from build123d import *

# Parameters (mm, degrees)
SKETCH1_W           = 80
SKETCH1_H           = 80
BOSS_EXTRUDE1_DEPTH = 5
SKETCH2_W           = 10
SKETCH2_H           = 4.637634929
BOSS_EXTRUDE2_DEPTH = 7
SKETCH3_R           = 1.5
CUT_EXTRUDE1_DEPTH  = 91


with BuildPart() as part:
    # Sketch1 → Boss-Extrude1 (new body)
    with BuildSketch(Plane.XY):
        Polygon((-50, 40), (-45, 40), (-45, 50), (45, 50), (45, 40), (50, 40), (50, -40), (45, -40), (45, -50), (-45, -50), (-45, -40), (-50, -40), align=None)
        Rectangle(SKETCH1_W, SKETCH1_H, mode=Mode.SUBTRACT)
    extrude(amount=BOSS_EXTRUDE1_DEPTH)

    # Sketch2 → Boss-Extrude2 (add)
    with BuildSketch(Plane.XY.offset(5)):
        with Locations((45, -37.681182535)):
            Rectangle(SKETCH2_W, SKETCH2_H)
        with Locations((-45, -37.681182535)):
            Rectangle(SKETCH2_W, SKETCH2_H)
        with Locations((-45, 37.681182535)):
            Rectangle(SKETCH2_W, SKETCH2_H)
        with Locations((45, 37.681182535)):
            Rectangle(SKETCH2_W, SKETCH2_H)
    extrude(amount=BOSS_EXTRUDE2_DEPTH)

    # Sketch3 → Cut-Extrude1 (cut, through all)
    with BuildSketch(Plane.XZ.offset(40)):
        with Locations((-47.5, 8)):
            Circle(SKETCH3_R)
        with Locations((47.5, 8)):
            Circle(SKETCH3_R)
    extrude(amount=-CUT_EXTRUDE1_DEPTH, mode=Mode.SUBTRACT)


solid = part.part
CAD build for the part. Positions are in the model's coordinates, mm. A direction names the side the tool comes from. Give positions to 0.01 mm unless a question says otherwise; leave off trailing zeros. Loops run counter-clockwise (first coordinate to the right, second up) from the corner with the lowest first, then second, coordinate; pieces in that order, holes last. Notation, with made-up numbers: M -29,62.5 L -15,62.5 A6 cw -15,67.5 Z; hole C 12.25,-7.5 d5. An arc over 180 degrees is marked long. One line per question, with ' | ' between items. Start each with the question number.
1. Probe L1, parallel to Z at x = 47.5, y = 36.75; L2, parallel to Y at x = -44, z = 7.5; L3, parallel to Y at x = 0, z = 2.25. List the from-to ranges inside material, lowest first. Write a range as from..to.
2. Two-plate mould, pull along X, no slides. Class faces 1 (the face through (45, 45, 2)), 2 (the face through (46, -38, 8)), 3 (the face through (46, 38, 8)), 4 (the face through (-45, -38, 12)): pulls with the +X half, pulls with the -X half, needs draft (parallel to the pull), parting line crosses it, or undercut.
3. Flat gauge pins, fed straight in: pin 1 (8 mm diameter, centred on x = 45.5, y = -4.5, fed in from +Z); pin 2 (5.5 mm diameter, centred on x = -45.5, z = 9, fed in from +Y); pin 3 (2.5 mm diameter, centred on x = -47.5, z = 8, fed in from +Y); pin 4 (3 mm diameter, centred on x = 44, z = 7, fed in from -Y). Where does each tip first touch, or does it go through?
4. Saw through at B-B on y = -38.5. Give the cut face in (x, z), plus the area to 3 significant figures.
5. Saw through at D-D on x = -32.5. Give the cut face in (y, z), plus the area to 3 significant figures.
6. Saw through at A-A on z = 8. State how many separate pieces and enclosed holes the cut face has, plus the area to 3 significant figures.
7. 3-axis set-ups, long thin cutter, end or side, ignore diameter. For faces 5 (the face through (45, -45, 2)), 6 (the face through (40, -1, 3)), 7 (the face through (-45, 0, 5)), 8 (the face through (-45, -45, 2)): which of +Z, -Z, +X, -X, +Y, -Y reach the whole face in a straight line?
8. Saw through at C-C on x = 47.5. Give the cut face in (y, z), plus the area to 3 significant figures.
Result sheet:
1) L1: z = 0..6.5, 9.5..12 | L2: y = -40..-35.36, 35.36..40 | L3: y = -50..-40, 40..50
2) face 1: pulls with the +X half | face 2: undercut | face 3: undercut | face 4: needs draft
3) pin 1: stops at z = 5 | pin 2: stops at y = 40 | pin 3: passes through | pin 4: stops at y = -40
4) outline: M -50,0 L -40,0 L -40,12 L -50,12 Z; M 40,0 L 50,0 L 50,12 L 40,12 Z; hole C -47.5,8 d3; hole C 47.5,8 d3 | area: 226 mm^2
5) outline: M -50,0 L -40,0 L -40,5 L -50,5 Z; M 40,0 L 50,0 L 50,5 L 40,5 Z | area: 100 mm^2
6) separate pieces: 8 | enclosed holes: 0 | area: 130 mm^2
7) face 5: +Z, -Z, +X, -Y | face 6: +Z, -Z | face 7: +Z, +X, -X | face 8: +Z, -Z, -X, -Y
8) outline: M -40,0 L 40,0 L 40,6.5 L 35.36,6.5 L 35.36,5 L -35.36,5 L -35.36,6.5 L -40,6.5 Z; M -40,9.5 L -35.36,9.5 L -35.36,12 L -40,12 Z; M 35.36,9.5 L 40,9.5 L 40,12 L 35.36,12 Z | area: 437 mm^2
